The drawing under review shows one solid part. Ordinate dimensions are in mm from its lowest x, y, z. A direction names the side the tool comes from. Round coordinates to 2 decimals unless told otherwise and drop trailing zeros. Order: outer loops, then holes, each group sorted by start corner. A loop starts at its lowest first (then second) coordinate and runs counter-clockwise, first axis right, second up. Notation, with made-up numbers: (74, 82.25) -> (106, 82.25) arc R31 ccw to (106, 111.25) -> close; hole circle Ø4 at (25.5, 74.5). An arc over 180 degrees is marked (long way). Use a Markdown table: item, result. Add a question column.
1) Consider section A-A (z = 4). State the section outline as (x, y) points, plus the area to 3 significant figures.
2) Consider section C-C (y = 18.75). State the section outline as (x, z) points.
3) Consider section B-B (x = 4). State the section outline as (y, z) points.
4) Machinability: for the marked faces 1 and 2, which of the approach directions +Z, -Z, +X, -X, +Y, -Y give a long, thin tool a straight path to every point of the face, cutting with its end or side? Answer none if there is none.
5) Clearance check with flat-ended pins moving along their axes: P1, Ø2, axis at x = 5, z = 4, coming from the -Y side; P2, Ø1, axis at y = 12.5, z = 6.5, coming from the +X side; P3, Ø1, axis at y = 7.5, z = 1, coming from the -X side; P4, Ø1.5, axis at x = 2.5, y = 11.5, coming from the +Z side. State where each tip first meets the part, or that it passes through.
6) Wall thickness on line 1 along Y through (x, z) = (2, 7); line 2 along Y through (x, z) = (3, 6.75); line 3 along X through (y, z) = (10, 6.75): over which ranges is each line inside the solid? List them lowest first. Write a range as [from, to].
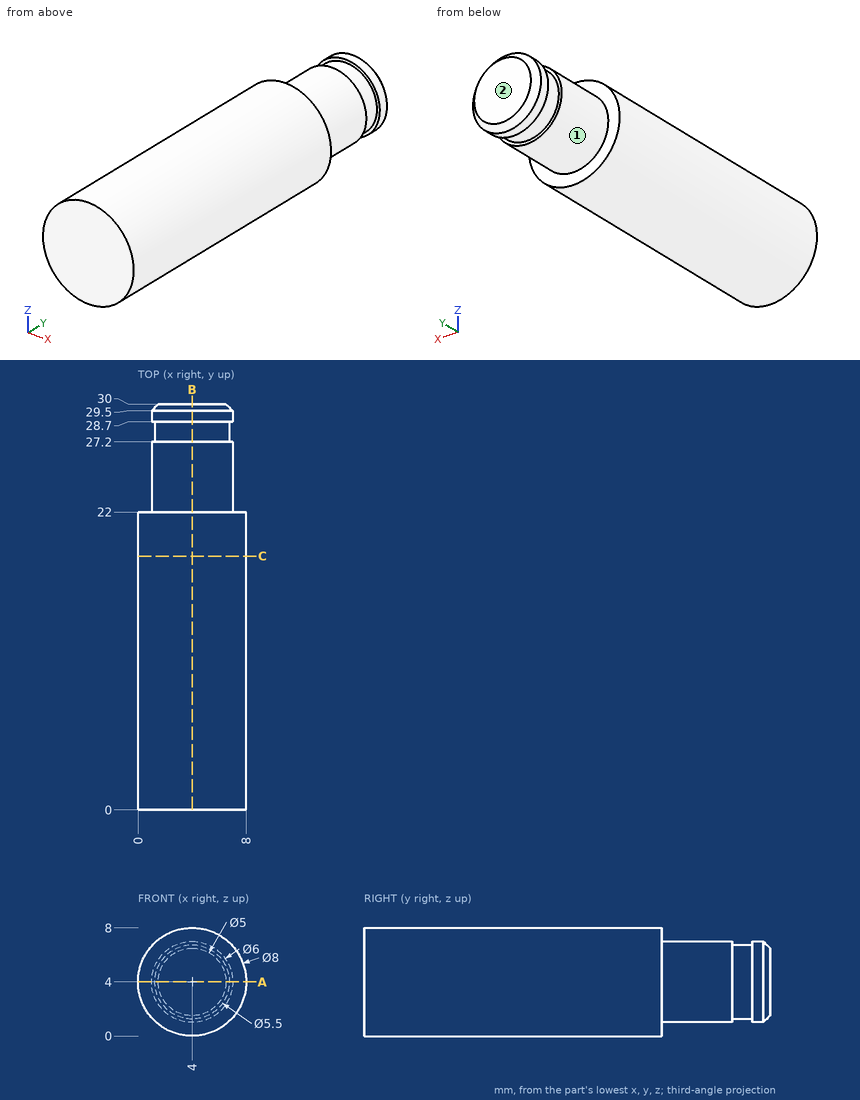
Results list:
| question | item | result |
|---|---|---|
| 1 | outline | (0, 0) -> (8, 0) -> (8, 22) -> (7, 22) -> (7, 27.2) -> (6.75, 27.2) -> (6.75, 28.7) -> (7, 28.7) -> (7, 29.5) -> (6.5, 30) -> (1.5, 30) -> (1, 29.5) -> (1, 28.7) -> (1.25, 28.7) -> (1.25, 27.2) -> (1, 27.2) -> (1, 22) -> (0, 22) -> close |
| 1 | area | 223 mm2 |
| 2 | outline | circle Ø8 at (4, 4) |
| 3 | outline | (0, 0) -> (22, 0) -> (22, 1) -> (27.2, 1) -> (27.2, 1.25) -> (28.7, 1.25) -> (28.7, 1) -> (29.5, 1) -> (30, 1.5) -> (30, 6.5) -> (29.5, 7) -> (28.7, 7) -> (28.7, 6.75) -> (27.2, 6.75) -> (27.2, 7) -> (22, 7) -> (22, 8) -> (0, 8) -> close |
| 4 | face 1 | +Y |
| 4 | face 2 | +Z, -Z, +X, -X, +Y |
| 5 | P1 | y = 0 |
| 5 | P2 | x = 7.46 |
| 5 | P3 | x = 0.88 |
| 5 | P4 | z = 7.93 |
| 6 | line 1 | [0, 22] |
| 6 | line 2 | [0, 27.2], [28.7, 29.57] |
| 6 | line 3 | [1.1, 6.9] |
